from build123d import *

# Parameters (mm, degrees)
BOSS_EXTRUDE1_DEPTH = 20
BOSS_EXTRUDE3_DEPTH = 10
SKETCH3_R           = 4.5
CUT_EXTRUDE1_DEPTH  = 32.393711542
CUT_EXTRUDE2_DEPTH  = 20
SKETCH5_R           = 3
CUT_EXTRUDE3_DEPTH  = 41
SKETCH6_R           = 4.25
CUT_EXTRUDE4_DEPTH  = 4
SKETCH7_R           = 4.25
CUT_EXTRUDE5_DEPTH  = 4


with BuildPart() as part:
    # Sketch1 → Boss-Extrude1 (new body)
    with BuildSketch(Plane(origin=(0, 0, 0), x_dir=(1, 0, 0), z_dir=(0, 1, 0))):
        Polygon((-10.75, 15), (-10.75, -6.5), (10.75, -6.5), (10.75, 15), (20, 15), (20, -15), (-20, -15), (-20, 15), align=None)
    extrude(amount=BOSS_EXTRUDE1_DEPTH)

    # Sketch2 → Boss-Extrude3 (add, symmetric)
    with BuildSketch(Plane(origin=(0, 0, 0), x_dir=(0, 0, -1), z_dir=(1, 0, 0))):
        Polygon((-15, 20), (-15, 0), (-46.393711542, 0), (-33.126155741, 28.452365235), align=None)
    extrude(amount=BOSS_EXTRUDE3_DEPTH, both=True)

    # Sketch3 → Cut-Extrude1 (cut, through all)
    with BuildSketch(Plane(origin=(0, 10.682542773, -4.981351504), x_dir=(1, 0, 0), z_dir=(0, 0.906307787, -0.422618262))):
        with Locations((0, -32.04698204)):
            Circle(SKETCH3_R)
    extrude(amount=-CUT_EXTRUDE1_DEPTH, mode=Mode.SUBTRACT)

    # Sketch4 → Cut-Extrude2 (cut)
    with BuildSketch(Plane(origin=(0, -10.162536328, 4.738868516), x_dir=(1, 0, 0), z_dir=(0, 0.906307787, -0.422618262))):
        Polygon((4.041451884, -39.04698204), (8.082903769, -32.04698204), (4.041451884, -25.04698204), (-4.041451884, -25.04698204), (-8.082903769, -32.04698204), (-4.041451884, -39.04698204), align=None)
    extrude(amount=-CUT_EXTRUDE2_DEPTH, mode=Mode.SUBTRACT)

    # Sketch5 → Cut-Extrude3 (cut, through all)
    with BuildSketch(Plane(origin=(20, 0, 0), x_dir=(0, 0, -1), z_dir=(1, 0, 0))):
        with Locations((4.5, 10)):
            Circle(SKETCH5_R)
    extrude(amount=-CUT_EXTRUDE3_DEPTH, mode=Mode.SUBTRACT)

    # Sketch6 → Cut-Extrude4 (cut)
    with BuildSketch(Plane(origin=(20, 0, 0), x_dir=(0, 0, -1), z_dir=(1, 0, 0))):
        with Locations((4.5, 10)):
            Circle(SKETCH6_R)
    extrude(amount=-CUT_EXTRUDE4_DEPTH, mode=Mode.SUBTRACT)

    # Sketch7 → Cut-Extrude5 (cut)
    with BuildSketch(Plane.ZY.offset(20)):
        with Locations((-4.5, 10)):
            Circle(SKETCH7_R)
    extrude(amount=-CUT_EXTRUDE5_DEPTH, mode=Mode.SUBTRACT)


solid = part.part
Source: CAD feature listing. Evaluate the final solid. Frame: model axes, mm. A direction names the side the tool comes from. Give positions to 0.01 mm unless a question says otherwise; leave off trailing zeros. Write each loop counter-clockwise with the first axis right and the second up, starting at its lowest first coordinate (ties: lowest second). Pieces come first, ordered by that corner, then holes. Notation, with made-up numbers: M 59.25,12 L 114.25,12 A19 cw 114.25,19 Z; hole C 87.25,21 d7. An arc over 180 degrees is marked long. Return JSON: item names as keys, results as strings. Group by question number.
1) Cut plane D-D, the plane x = 14.5. Output: boundary loops of the cut face in (y, z), plus the area to 3 significant figures.
2) Cut plane B-B, the plane x = 2. Output: boundary loops of the cut face in (y, z).
3) Set-up query: faces 1 (the face through (0, 20, 10)), 2 (the face through (-10, 11, 27)), 3 (the face through (-18.03, 7.41, -7.87)), 4 (the face through (10.75, 8, -2)), 5 (the face through (15, 10, 15)). Return all of +Z, -Z, +X, -X, +Y, -Y with unobstructed straight access to the full face (end or side cutting, diameter ignored); none if empty.
4) Cut plane A-A, the plane z = -4.5. Output: boundary loops of the cut face in (x, y), plus the area to 3 significant figures.
5) Pin query (flat end, axial travel): P1, Ø5, axis at x = -17, y = 13.5, coming from the +Z side; P2, Ø24, axis at x = -1, z = -5.5, coming from the +Y side; P3, Ø6, axis at x = 4, y = 5, coming from the -Z side; P4, Ø3.5, axis at y = 10, z = -4.5, coming from the -X side. Return the tip coordinate at first contact, or that it passes through.
6) Cut plane C-C, the plane y = 10. Give the number of separate pieces and of enclosed holes in the cut face, plus the area to 3 significant figures.
7) Pull-direction query (X, two-part tool) for faces 6 (the face through (20, 10, 0)), 7 (the face through (13.4, 10.1, -1.5)), 8 (the face through (-0.057, 3.214, 41.585)); classes: pulls with the +X half, pulls with the -X half, needs draft (parallel to the pull), parting line crosses it, or undercut.
8) Material intervals for line 1 along X through (y, z) = (17.75, -4); line 2 along X through (y, z) = (13, -6.5); line 3 along Y through (x, z) = (13.75, -4.5), sorted ascending. Write a range as [from, to].
Recorded:
{
 "1": {"outline": "M 0,-15 L 20,-15 L 20,15 L 0,15 Z; hole C 10,-4.5 d6", "area": "572 mm²"},
 "2": {"outline": "M 0,6.5 L 20,6.5 L 20,15 L 22.52,20.41 L 1.68,30.13 L 0.42,27.44 L 0,27.64 Z; M 0,43.08 L 6.34,40.13 L 5.08,37.44 L 25.93,27.72 L 28.45,33.13 L 0,46.39 Z"},
 "3": {"face 1": "-Z, +X, -X, +Y", "face 2": "+Z, -X, +Y, -Y", "face 3": "-X", "face 4": "-Z, +Y, -Y", "face 5": "+Z, +X, +Y, -Y"},
 "4": {"outline": "M -20,0 L -10.75,0 L -10.75,7 L -16,7 L -16,5.75 L -20,5.75 Z; M -20,14.25 L -16,14.25 L -16,13 L -10.75,13 L -10.75,20 L -20,20 Z; M 10.75,0 L 20,0 L 20,5.75 L 16,5.75 L 16,7 L 10.75,7 Z; M 10.75,13 L 16,13 L 16,14.25 L 20,14.25 L 20,20 L 10.75,20 Z", "area": "239 mm²"},
 "5": {"P1": "stops at z = 15", "P2": "stops at y = 20", "P3": "stops at z = 6.5", "P4": "passes through"},
 "6": {"separate pieces": "3", "enclosed holes": "1", "area": "1,070 mm²"},
 "7": {"face 6": "pulls with the +X half", "face 7": "needs draft", "face 8": "undercut"},
 "8": {"line 1": "x = [-20, -10.75], [10.75, 20]", "line 2": "x = [-16, -10.75], [10.75, 16]", "line 3": "y = [0, 7], [13, 20]"}
}
